from build123d import *

# Parameters (mm, degrees)
F0_W     = 30
F0_H     = 18
F1_DEPTH = 3
F2_R     = 3
F3_R     = 1.55
F3_R_2   = 10
F4_DEPTH = 3.001


with BuildPart() as f1:
    # F0 (on Front) → F1 (new body)
    with BuildSketch(Plane.XZ):
        Polygon((-21.75, -10), (-21.75, -35), (21.75, -35), (21.75, -10), (26.25, -10), (26.25, 35), (-26.25, 35), (-26.25, -10), align=None)
        with Locations((0, -19)):
            Rectangle(F0_W, F0_H, mode=Mode.SUBTRACT)
    extrude(amount=F1_DEPTH)

    # F2
    f2_edges = [f1.edges().sort_by_distance(p)[0] for p in [
        (-15, -1.5, -28),
        (15, -1.5, -28),
        (15, -1.5, -10),
        (-15, -1.5, -10),
    ]]
    fillet(f2_edges, radius=F2_R)

    # F3 (on face) → F4 (cut, through all)
    with BuildSketch(Plane.XZ.offset(3)):
        with Locations((-9, 24.5)):
            Circle(F3_R)
        with Locations((15, 24.5)):
            Circle(F3_R)
        with Locations((-9, 0.5)):
            Circle(F3_R)
        with Locations((15, 0.5)):
            Circle(F3_R)
        with Locations((3, 12.5)):
            Circle(F3_R_2)
    extrude(amount=-F4_DEPTH, mode=Mode.SUBTRACT)


solid = f1.part
Geometry: final body of the model. Coordinates: model frame, mm. A direction names the side the tool comes from. Give positions to 0.01 mm unless a question says otherwise; leave off trailing zeros. Write each loop counter-clockwise with the first axis right and the second up, starting at its lowest first coordinate (ties: lowest second). Pieces come first, ordered by that corner, then holes. Notation, with made-up numbers: (78.5, -3.5) -> (116.5, -3.5) arc R10 ccw to (116.5, 2.5) -> close; hole circle Ø6 at (-40, 82). An arc over 180 degrees is marked (long way). Answer in a Markdown table with one row per item.
(1) Draft query along X for faces 4 (the cylindrical face through (14.798, -1.521, 26.037)), 5 (the flat face through (21.75, -1, -23)), 6 (the flat face through (0, 0, 0)). Return one class per face: +X half, -X half, draft (parallel to the pull), parting line (faces both ways), or undercut.
Answers below:
| item | result |
|---|---|
| face 4 | undercut |
| face 5 | +X half |
| face 6 | draft |
(2) Ray query, line 1 along Z through (x, y) = (-9, -2.2); line 2 along Z through (x, y) = (3, -1.85); line 3 along X through (y, z) = (-1.3, -23.5). Return the intervals inside material, ascending. Write a range as [from, to].
Answers below:
| item | result |
|---|---|
| line 1 | [-35, -28], [-10, -1.05], [2.05, 22.95], [26.05, 35] |
| line 2 | [-35, -28], [-10, 2.5], [22.5, 35] |
| line 3 | [-21.75, -15], [15, 21.75] |
(3) Pin query (flat end, axial travel): pin 1 (0.9 mm diameter, centred on y = -2, z = -19, fed in from -X); pin 2 (0.9 mm diameter, centred on y = -2, z = -18.5, fed in from +X); pin 3 (5 mm diameter, centred on x = -17, z = -12, fed in from +Y); pin 4 (1.5 mm diameter, centred on x = -25, y = -1, fed in from -Z). Return the tip coordinate at first contact, or that it passes through.
Answers below:
| item | result |
|---|---|
| pin 1 | x = -21.75 |
| pin 2 | x = 21.75 |
| pin 3 | y = 0 |
| pin 4 | z = -10 |
(4) Set-up query: faces 1 (the flat face through (15, -1, -19)), 2 (the flat face through (-24, -1, -10)), 3 (the flat face through (24, -1, -10)). Return all of +Z, -Z, +X, -X, +Y, -Y with unobstructed straight access to the full face (end or side cutting, diameter ignored); none if empty.
Answers below:
| item | result |
|---|---|
| face 1 | +Y, -Y |
| face 2 | -Z, -X, +Y, -Y |
| face 3 | -Z, +X, +Y, -Y |
(5) Section query D-D on z = 12.5. Return loops of the section in (x, y), then the cut area to 3 significant figures.
Answers below:
| item | result |
|---|---|
| outline | (-26.25, -3) -> (-7, -3) -> (-7, 0) -> (-26.25, 0) -> close; (13, -3) -> (26.25, -3) -> (26.25, 0) -> (13, 0) -> close |
| area | 97.5 mm^2 |
(6) Section query B-B on y = -0.7. Return loops of the section in (x, z), then the cut area to 3 significant figures.
Answers below:
| item | result |
|---|---|
| outline | (-26.25, -10) -> (-21.75, -10) -> (-21.75, -35) -> (21.75, -35) -> (21.75, -10) -> (26.25, -10) -> (26.25, 35) -> (-26.25, 35) -> close; hole (-15, -25) arc R3 ccw to (-12, -28) -> (12, -28) arc R3 ccw to (15, -25) -> (15, -13) arc R3 ccw to (12, -10) -> (-12, -10) arc R3 ccw to (-15, -13) -> close; hole circle Ø3.1 at (-9, 0.5); hole circle Ø3.1 at (-9, 24.5); hole circle Ø20 at (3, 12.5); hole circle Ø3.1 at (15, 0.5); hole circle Ø3.1 at (15, 24.5) |
| area | 2,570 mm^2 |
(7) Section query A-A on x = -9. Return loops of the section in (y, z).
Answers below:
| item | result |
|---|---|
| outline | (-3, -35) -> (0, -35) -> (0, -28) -> (-3, -28) -> close; (-3, -10) -> (0, -10) -> (0, -1.05) -> (-3, -1.05) -> close; (-3, 2.05) -> (0, 2.05) -> (0, 22.95) -> (-3, 22.95) -> close; (-3, 26.05) -> (0, 26.05) -> (0, 35) -> (-3, 35) -> close |
(8) Section query C-C on z = 0.5. Return loops of the section in (x, y), then the cut area to 3 significant figures.
Answers below:
| item | result |
|---|---|
| outline | (-26.25, -3) -> (-10.55, -3) -> (-10.55, 0) -> (-26.25, 0) -> close; (-7.45, -3) -> (13.45, -3) -> (13.45, 0) -> (-7.45, 0) -> close; (16.55, -3) -> (26.25, -3) -> (26.25, 0) -> (16.55, 0) -> close |
| area | 139 mm^2 |
